Can you work these out from the model? Positions are in its coordinate system, mm. A direction names the side the tool comes from. Round coordinates to 2 decimals unless told otherwise and drop trailing zeros. Loops run counter-clockwise (first coordinate to the right, second up) from the corner with the lowest first, then second, coordinate; pieces in that order, holes last. Notation, with made-up numbers: M 77,30.5 L 116,30.5 A26 cw 116,44.5 Z; hole C 41.5,67 d5. An arc over 180 degrees is marked long. Return JSON: item names as keys, results as strings.
```python
from build123d import *

# Parameters (mm, degrees)
CROQUIS1_R                 = 20.5
SALIENTE_EXTRUIR1_DEPTH    = 3.5
CORTAR_EXTRUIR2_DEPTH      = 3
CORTAR_EXTRUIR2_DEPTH_BACK = 10
CROQUIS3_W                 = 4
CROQUIS3_H                 = 1.5
CROQUIS4_R                 = 19.5
CORTAR_EXTRUIR3_DEPTH      = 3
CROQUIS5_R                 = 19
CORTAR_EXTRUIR4_DEPTH      = 3
REDONDEO1_R                = 1.5


with BuildPart() as part:
    # Croquis1 → Saliente-Extruir1 (new body)
    with BuildSketch(Plane.XY):
        Circle(CROQUIS1_R)
    extrude(amount=SALIENTE_EXTRUIR1_DEPTH)

    # Croquis3 → Cortar-Extruir2 (cut, two sides: drawn at the far end of the back side and taken through both)
    with BuildSketch(Plane(origin=(0, 20, 0), x_dir=(-1, 0, 0), z_dir=(0, 1, 0)).offset(-CORTAR_EXTRUIR2_DEPTH_BACK)):
        with Locations((0, 0.75)):
            Rectangle(CROQUIS3_W, CROQUIS3_H)
    extrude(amount=CORTAR_EXTRUIR2_DEPTH + CORTAR_EXTRUIR2_DEPTH_BACK, mode=Mode.SUBTRACT)

    # Croquis4 → Cortar-Extruir3 (cut)
    with BuildSketch(Plane(origin=(0, 0, 0), x_dir=(-1, 0, 0), z_dir=(0, 0, -1))):
        Circle(CROQUIS4_R)
    extrude(amount=-CORTAR_EXTRUIR3_DEPTH, mode=Mode.SUBTRACT)

    # Croquis5 → Cortar-Extruir4 (cut)
    with BuildSketch(Plane(origin=(0, 0, 3), x_dir=(-1, 0, 0), z_dir=(0, 0, -1))):
        Circle(CROQUIS5_R)
    extrude(amount=-CORTAR_EXTRUIR4_DEPTH, mode=Mode.SUBTRACT)

    # Redondeo1
    redondeo1_edges = [part.edges().sort_by_distance(p)[0] for p in [
        (-20.5, 0, 3.5),
    ]]
    fillet(redondeo1_edges, radius=REDONDEO1_R - 0.0001)  # a hair under: the kernel refuses the full size


solid = part.part
```
Q1. Thinking about a two-plate mould opening in X: for faces 3 (the flat face through (0, -20, 0)), 4 (the cylindrical face through (-4.444, -20.013, 0.986)), 5 (the cylindrical face through (-8.767, -16.856, 3.246)), which applies, pulls with the +X half, pulls with the -X half, needs draft (parallel to the pull), parting line crosses it, or undercut?
Results:
{"face 3": "needs draft", "face 4": "parting line crosses it", "face 5": "undercut"}
Q2. I'm going to push flat-ended pins straight in: pin 1 Ø0.9 at (x, y) = (0, 20) entering from -Z; pin 2 Ø6 at (x, y) = (-13.5, -3.5) entering from -Z; pin 3 Ø1.1 at (y, z) = (19.5, 0.5) entering from +X; pin 4 Ø2 at (x, z) = (10.5, 0.5) entering from +Y. Where does each tip first touch, or does it pass through?
Results:
{"pin 1": "stops at z = 1.5", "pin 2": "passes through", "pin 3": "stops at x = 7.82", "pin 4": "stops at y = 18.17"}
Q3. On a 3-axis mill with a long thin cutter (end or side, diameter ignored), from which of +Z, -Z, +X, -X, +Y, -Y can I reach the whole of each face in a straight line? I mean faces 1 (the cylindrical face through (2.539, 19.334, 1.479)), 2 (the flat face through (2, 20, 1)). Say none if no direction works.
Results:
{"face 1": "-Z", "face 2": "-Z, +Y"}
Q4. If I drill on line 1 along X through (y, z) = (0, 1.05); line 2 along Y through (x, z) = (-12.5, 2.85), over which ranges is the centre line in solid material (lowest first)?
Results:
{"line 1": "x = -20.5 to -19.5, 19.5 to 20.5", "line 2": "y = -15.91 to -14.97, 14.97 to 15.91"}
Q5. Suppose I cut it at C-C, the plane z = 0.95. Please give me the cut outline in (x, y).
Results:
{"outline": "M -2,19.4 L -2,20.4 A20.5 ccw long 2,20.4 L 2,19.4 A19.5 cw long Z"}
